Could you check a few things on this model? Use its own coordinates, in mm. Round coordinates to 2 decimals unless told otherwise and drop trailing zeros. Loops run counter-clockwise (first coordinate to the right, second up) from the corner with the lowest first, then second, coordinate; pieces in that order, holes last. Notation, with made-up numbers: (51, -14) -> (101, -14) arc R20 cw to (101, 10) -> close; hole circle Ø10 at (-22, 58). An arc over 180 degrees is marked (long way). Put each result on its own line as item: value. Start each with the question number.
1. Imagine slicing it at C-C, the plane x = -35. Please give me the cut outline in (y, z).
2. Imagine slicing it at A-A, the plane x = 0. Please give me the cut outline in (y, z), and give its area (3 significant figures).
3. Imagine slicing it at B-B, the plane y = 0. Please give me the cut outline in (x, z), and give its area (3 significant figures).
4. I need wall thicknesses on line 1 (Y direction, x = -35, z = 2.75); line 2 (X direction, y = -45.5, z = 2.5); line 3 (X direction, y = 90.5, z = 0.5). Which ranges of each line are inside material? Lowest first, please. Write a range as [from, to].
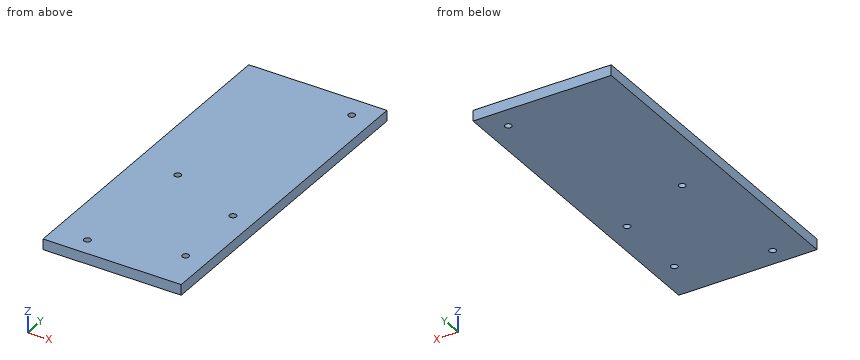
```python
from build123d import *

# Parameters (mm, degrees)
F0_W     = 200
F0_H     = 200
F1_DEPTH = 5
F2_R     = 1.5875
F3_DEPTH = 5.001
F4_R     = 1.5875
F5_DEPTH = 25


with BuildPart() as f1:
    # F0 (on Top) → F1 (new body)
    with BuildSketch(Plane.XY):
        Rectangle(F0_W, F0_H)
    extrude(amount=F1_DEPTH)

    # F2 (on face) → F3 (cut, through all)
    with BuildSketch(Plane.XY.offset(5)):
        Circle(F2_R)
        with Locations((0, -35.65053)):
            Circle(F2_R)
        with Locations((-39.612573, -46.225714)):
            Circle(F2_R)
        with Locations((-35, 14.476054)):
            Circle(F2_R)
        with Locations((0, 89.476054)):
            Circle(F2_R)
    extrude(amount=-F3_DEPTH, mode=Mode.SUBTRACT)

    # F4 (on face) → F5 (cut)
    with BuildSketch(Plane.XY.offset(5)):
        Polygon((-55, -55), (-55, 100), (-100, 100), (-100, -100), (100, -100), (100, 100), (10, 100), (10, -55), align=None)
        Circle(F4_R)
        with Locations((0, -35.65053)):
            Circle(F4_R)
        with Locations((-39.612573, -46.225714)):
            Circle(F4_R)
        with Locations((-35, 14.476054)):
            Circle(F4_R)
        with Locations((0, 89.476054)):
            Circle(F4_R)
    extrude(amount=-F5_DEPTH, mode=Mode.SUBTRACT)


solid = f1.part
```
Entries:
1. outline: (-55, 0) -> (12.89, 0) -> (12.89, 5) -> (-55, 5) -> close; (16.06, 0) -> (100, 0) -> (100, 5) -> (16.06, 5) -> close
2. outline: (-55, 0) -> (-37.24, 0) -> (-37.24, 5) -> (-55, 5) -> close; (-34.06, 0) -> (-1.59, 0) -> (-1.59, 5) -> (-34.06, 5) -> close; (1.59, 0) -> (87.89, 0) -> (87.89, 5) -> (1.59, 5) -> close; (91.06, 0) -> (100, 0) -> (100, 5) -> (91.06, 5) -> close
2. area: 727 mm^2
3. outline: (-55, 0) -> (-1.59, 0) -> (-1.59, 5) -> (-55, 5) -> close; (1.59, 0) -> (10, 0) -> (10, 5) -> (1.59, 5) -> close
3. area: 309 mm^2
4. line 1: [-55, 12.89], [16.06, 100]
4. line 2: [-55, -41.02], [-38.2, 10]
4. line 3: [-55, -1.21], [1.21, 10]
